```python
from build123d import *

# Parameters (mm, degrees)
BASE_DEPTH                   = 6.35
SUPPORT_CUTOUTS_REACH        = 181.717
SKETCH4_W                    = 12.7
SKETCH4_H                    = 6.35
SUPPORT_CUTOUT_PATTERN_COUNT = 4
F_8_CLEARANCE_HOLE1_D        = 4.4958
CABLE_HOLES_REACH            = 181.717
SKETCH14_R                   = 7.9375
ALIGNER_MOUNTING_HOLES_D     = 4.3053
CIRPATTERN1_COUNT            = 4
CUT_EXTRUDE2_DEPTH           = 180.717340566
CUT_EXTRUDE3_DEPTH           = 180.717340566


with BuildPart() as part:
    # Base sketch → Base (new body)
    with BuildSketch(Plane(origin=(0, 0, 0), x_dir=(1, 0, 0), z_dir=(0, 1, 0))):
        Polygon((-127, 52.605122421), (-127, -52.605122421), (-52.605122421, -127), (52.605122421, -127), (127, -52.605122421), (127, 52.605122421), (52.605122421, 127), (-52.605122421, 127), align=None)
    extrude(amount=BASE_DEPTH)

    # Sketch4 → Support cutouts (cut, up to next)
    with BuildSketch(Plane(origin=(0, 6.35, 0), x_dir=(1, 0, 0), z_dir=(0, 1, 0)), mode=Mode.PRIVATE) as support_cutouts_sk1:
        with Locations((0, 73.025)):
            Rectangle(SKETCH4_W, SKETCH4_H)
    support_cutouts_tool1 = extrude(support_cutouts_sk1.sketch, amount=-SUPPORT_CUTOUTS_REACH, mode=Mode.PRIVATE) & part.part
    support_cutouts = support_cutouts_tool1.solids().sort_by_distance((0, 6.35, -73.025))[0]
    add(support_cutouts, mode=Mode.SUBTRACT)

    # Support cutout pattern: Support cutouts ×4 about axis
    support_cutout_pattern_axis = Axis((0, 0, 0), (0, 1, 0))
    for i in range(1, SUPPORT_CUTOUT_PATTERN_COUNT):
        add(support_cutouts.rotate(support_cutout_pattern_axis, i * 360 / SUPPORT_CUTOUT_PATTERN_COUNT), mode=Mode.SUBTRACT)

    # 8 Clearance Hole1 (through all)
    with Locations(Plane(origin=(0, 6.35, 0), x_dir=(1, 0, 0), z_dir=(0, 1, 0))):
        with Locations((-82.55, 34.193329574), (-34.193329574, 82.55), (34.193329574, 82.55), (82.55, 34.193329574), (82.55, -34.193329574), (34.193329574, -82.55), (-34.193329574, -82.55), (-82.55, -34.193329574)):
            Hole(F_8_CLEARANCE_HOLE1_D / 2)

    # Sketch14 → Cable holes (cut, up to next)
    with BuildSketch(Plane(origin=(0, 6.35, 0), x_dir=(1, 0, 0), z_dir=(0, 1, 0)), mode=Mode.PRIVATE) as cable_holes_sk1:
        with Locations(Location((-53.881536726, 53.881536726, 0), (0, 0, 270))):
            Circle(SKETCH14_R)
    cable_holes_tool1 = extrude(cable_holes_sk1.sketch, amount=-CABLE_HOLES_REACH, mode=Mode.PRIVATE) & part.part
    # Sketch14 → Cable holes (cut, up to next)
    with BuildSketch(Plane(origin=(0, 6.35, 0), x_dir=(1, 0, 0), z_dir=(0, 1, 0)), mode=Mode.PRIVATE) as cable_holes_sk2:
        with Locations(Location((53.881536726, 53.881536726, 0), (0, 0, 270))):
            Circle(SKETCH14_R)
    cable_holes_tool2 = extrude(cable_holes_sk2.sketch, amount=-CABLE_HOLES_REACH, mode=Mode.PRIVATE) & part.part
    # Sketch14 → Cable holes (cut, up to next)
    with BuildSketch(Plane(origin=(0, 6.35, 0), x_dir=(1, 0, 0), z_dir=(0, 1, 0)), mode=Mode.PRIVATE) as cable_holes_sk3:
        with Locations(Location((53.881536726, -53.881536726, 0), (0, 0, 270))):
            Circle(SKETCH14_R)
    cable_holes_tool3 = extrude(cable_holes_sk3.sketch, amount=-CABLE_HOLES_REACH, mode=Mode.PRIVATE) & part.part
    # Sketch14 → Cable holes (cut, up to next)
    with BuildSketch(Plane(origin=(0, 6.35, 0), x_dir=(1, 0, 0), z_dir=(0, 1, 0)), mode=Mode.PRIVATE) as cable_holes_sk4:
        with Locations(Location((-53.881536726, -53.881536726, 0), (0, 0, 270))):
            Circle(SKETCH14_R)
    cable_holes_tool4 = extrude(cable_holes_sk4.sketch, amount=-CABLE_HOLES_REACH, mode=Mode.PRIVATE) & part.part
    add(cable_holes_tool1.solids().sort_by_distance((-53.881537, 6.35, -53.881537))[0], mode=Mode.SUBTRACT)
    add(cable_holes_tool2.solids().sort_by_distance((53.881537, 6.35, -53.881537))[0], mode=Mode.SUBTRACT)
    add(cable_holes_tool3.solids().sort_by_distance((53.881537, 6.35, 53.881537))[0], mode=Mode.SUBTRACT)
    add(cable_holes_tool4.solids().sort_by_distance((-53.881537, 6.35, 53.881537))[0], mode=Mode.SUBTRACT)

    # aligner mounting holes (through all)
    with Locations(Plane(origin=(0, 6.35, 0), x_dir=(1, 0, 0), z_dir=(0, 1, 0))):
        with Locations((121.233457634, 40.411152545), (40.411152545, 121.233457634)):
            aligner_mounting_holes = Hole(ALIGNER_MOUNTING_HOLES_D / 2)

    # CirPattern1: aligner mounting holes ×4 about axis
    cirpattern1_axis = Axis((0, 0, 0), (0, 1, 0))
    for i in range(1, CIRPATTERN1_COUNT):
        add(aligner_mounting_holes.rotate(cirpattern1_axis, i * 360 / CIRPATTERN1_COUNT), mode=Mode.SUBTRACT)

    # Sketch28 → Cut-Extrude2 (cut, through all)
    with BuildSketch(Plane(origin=(0, 6.35, 0), x_dir=(1, 0, 0), z_dir=(0, 1, 0))):
        with BuildLine():
            Line((55.651152545, 80.367817332), (55.651152545, 107.308585695))
            ThreePointArc((55.651152545, 107.308585695), (57.611132647, 110.241903211), (61.071216575, 109.553649725))
            Line((61.071216575, 109.553649725), (109.553649725, 61.071216575))
            ThreePointArc((109.553649725, 61.071216575), (110.241903211, 57.611132647), (107.308585695, 55.651152545))
            Line((107.308585695, 55.651152545), (80.367817332, 55.651152545))
            ThreePointArc((80.367817332, 55.651152545), (79.152797434, 55.892835029), (78.122753301, 56.581088515))
            Line((78.122753301, 56.581088515), (56.581088515, 78.122753301))
            ThreePointArc((56.581088515, 78.122753301), (55.892835029, 79.152797434), (55.651152545, 80.367817332))
        make_face()
        with BuildLine():
            Line((80.367817332, -55.651152545), (107.308585695, -55.651152545))
            ThreePointArc((107.308585695, -55.651152545), (110.241903211, -57.611132647), (109.553649725, -61.071216575))
            Line((109.553649725, -61.071216575), (61.071216575, -109.553649725))
            ThreePointArc((61.071216575, -109.553649725), (57.611132647, -110.241903211), (55.651152545, -107.308585695))
            Line((55.651152545, -107.308585695), (55.651152545, -80.367817332))
            ThreePointArc((55.651152545, -80.367817332), (55.892835029, -79.152797434), (56.581088515, -78.122753301))
            Line((56.581088515, -78.122753301), (78.122753301, -56.581088515))
            ThreePointArc((78.122753301, -56.581088515), (79.152797434, -55.892835029), (80.367817332, -55.651152545))
        make_face()
        with BuildLine():
            Line((-55.651152545, -80.367817332), (-55.651152545, -107.308585695))
            ThreePointArc((-55.651152545, -107.308585695), (-57.611132647, -110.241903211), (-61.071216575, -109.553649725))
            Line((-61.071216575, -109.553649725), (-109.553649725, -61.071216575))
            ThreePointArc((-109.553649725, -61.071216575), (-110.241903211, -57.611132647), (-107.308585695, -55.651152545))
            Line((-107.308585695, -55.651152545), (-80.367817332, -55.651152545))
            ThreePointArc((-80.367817332, -55.651152545), (-79.152797434, -55.892835029), (-78.122753301, -56.581088515))
            Line((-78.122753301, -56.581088515), (-56.581088515, -78.122753301))
            ThreePointArc((-56.581088515, -78.122753301), (-55.892835029, -79.152797434), (-55.651152545, -80.367817332))
        make_face()
        with BuildLine():
            Line((-56.581088515, 78.122753301), (-78.122753301, 56.581088515))
            ThreePointArc((-78.122753301, 56.581088515), (-79.152797434, 55.892835029), (-80.367817332, 55.651152545))
            Line((-80.367817332, 55.651152545), (-107.308585695, 55.651152545))
            ThreePointArc((-107.308585695, 55.651152545), (-110.241903211, 57.611132647), (-109.553649725, 61.071216575))
            Line((-109.553649725, 61.071216575), (-61.071216575, 109.553649725))
            ThreePointArc((-61.071216575, 109.553649725), (-57.611132647, 110.241903211), (-55.651152545, 107.308585695))
            Line((-55.651152545, 107.308585695), (-55.651152545, 80.367817332))
            ThreePointArc((-55.651152545, 80.367817332), (-55.892835029, 79.152797434), (-56.581088515, 78.122753301))
        make_face()
    extrude(amount=-CUT_EXTRUDE2_DEPTH, mode=Mode.SUBTRACT)

    # Sketch29 → Cut-Extrude3 (cut, through all)
    with BuildSketch(Plane(origin=(0, 6.35, 0), x_dir=(1, 0, 0), z_dir=(0, 1, 0))):
        with BuildLine():
            Line((15.24, -2.2225), (15.24, 2.2225))
            ThreePointArc((15.24, 2.2225), (15.983948776, 4.018551224), (17.78, 4.7625))
            Line((17.78, 4.7625), (19.05, 4.7625))
            ThreePointArc((19.05, 4.7625), (20.846051224, 4.018551224), (21.59, 2.2225))
            Line((21.59, 2.2225), (21.59, -2.2225))
            ThreePointArc((21.59, -2.2225), (20.846051224, -4.018551224), (19.05, -4.7625))
            Line((19.05, -4.7625), (17.78, -4.7625))
            ThreePointArc((17.78, -4.7625), (15.983948776, -4.018551224), (15.24, -2.2225))
        make_face()
        with BuildLine():
            Line((2.2225, 15.24), (-2.2225, 15.24))
            ThreePointArc((-2.2225, 15.24), (-4.018551224, 15.983948776), (-4.7625, 17.78))
            Line((-4.7625, 17.78), (-4.7625, 19.05))
            ThreePointArc((-4.7625, 19.05), (-4.018551224, 20.846051224), (-2.2225, 21.59))
            Line((-2.2225, 21.59), (2.2225, 21.59))
            ThreePointArc((2.2225, 21.59), (4.018551224, 20.846051224), (4.7625, 19.05))
            Line((4.7625, 19.05), (4.7625, 17.78))
            ThreePointArc((4.7625, 17.78), (4.018551224, 15.983948776), (2.2225, 15.24))
        make_face()
        with BuildLine():
            Line((-2.2225, -15.24), (2.2225, -15.24))
            ThreePointArc((2.2225, -15.24), (4.018551224, -15.983948776), (4.7625, -17.78))
            Line((4.7625, -17.78), (4.7625, -19.05))
            ThreePointArc((4.7625, -19.05), (4.018551224, -20.846051224), (2.2225, -21.59))
            Line((2.2225, -21.59), (-2.2225, -21.59))
            ThreePointArc((-2.2225, -21.59), (-4.018551224, -20.846051224), (-4.7625, -19.05))
            Line((-4.7625, -19.05), (-4.7625, -17.78))
            ThreePointArc((-4.7625, -17.78), (-4.018551224, -15.983948776), (-2.2225, -15.24))
        make_face()
        with BuildLine():
            Line((-15.24, 2.2225), (-15.24, -2.2225))
            ThreePointArc((-15.24, -2.2225), (-15.983948776, -4.018551224), (-17.78, -4.7625))
            Line((-17.78, -4.7625), (-19.05, -4.7625))
            ThreePointArc((-19.05, -4.7625), (-20.846051224, -4.018551224), (-21.59, -2.2225))
            Line((-21.59, -2.2225), (-21.59, 2.2225))
            ThreePointArc((-21.59, 2.2225), (-20.846051224, 4.018551224), (-19.05, 4.7625))
            Line((-19.05, 4.7625), (-17.78, 4.7625))
            ThreePointArc((-17.78, 4.7625), (-15.983948776, 4.018551224), (-15.24, 2.2225))
        make_face()
    extrude(amount=-CUT_EXTRUDE3_DEPTH, mode=Mode.SUBTRACT)


solid = part.part
```
Geometry check sheet. Reference: the model listing, model coordinates, mm. A direction names the side the tool comes from. Round coordinates to 2 decimals unless told otherwise and drop trailing zeros. Order: outer loops, then holes, each group sorted by start corner. A loop starts at its lowest first (then second) coordinate and runs counter-clockwise, first axis right, second up. Notation, with made-up numbers: (34, 46.5) - (42, 46.5) arc R11 ccw to (42, 67.5) - close; hole circle Ø5 at (83, 51.5). An arc over 180 degrees is marked (long way). Use a Markdown table: item, result. Add a question column.
1) Gauge pin test, flat ends, axial feed: P1, Ø1.9, axis at x = -71.5, y = 3.5, coming from the +Z side; P2, Ø1, axis at x = 77, y = 4, coming from the -Z side; P3, Ø1.9, axis at y = 4, z = -73, coming from the +X side. Record the tip position at first contact, or that the pin passes through.
2) Section check B-B (y = 3.75). Count the separate pieces of the cut face and the enclosed holes in it, then the cut area to 3 significant figures.
3) Mould release check, pull along X, two halves, no side actions. Record for faces 1 (the flat face through (-6.35, 3, 73)), 2 (the flat face through (90.323, 3.131, -89.282)), 3 (the flat face through (84.973, 3.219, -85.652)): released by +X, released by -X, zero draft, split by the parting line, or undercut.
4) Set-up check for faces 4 (the flat face through (89.282, 3.131, 90.323)), 5 (the flat face through (0, 3, 76.2)): record each of +Z, -Z, +X, -X, +Y, -Y from which the full face is reachable in a straight line by a thin tool's end or side.
5) Thickness scan on line 1 along Z through (x, y) = (6, 1); line 2 along Z through (x, y) = (1, 0.75); line 3 along X through (y, z) = (3.5, 70.5). Record the ranges inside material, lowest first.
6) Section check A-A (x = -95). Record the cut outline in (y, z), then the cut area to 3 significant figures.
Established:
| question | item | result |
|---|---|---|
| 1 | P1 | z = 109.06 |
| 1 | P2 | z = -103.11 |
| 1 | P3 | x = 107.56 |
| 2 | separate pieces | 1 |
| 2 | enclosed holes | 32 |
| 2 | area | 46,000 mm2 |
| 3 | face 1 | undercut |
| 3 | face 2 | released by +X |
| 3 | face 3 | undercut |
| 4 | face 4 | +Z, +X, +Y, -Y |
| 4 | face 5 | +Y, -Y |
| 5 | line 1 | -127 to -76.2, -69.85 to 69.85, 76.2 to 127 |
| 5 | line 2 | -127 to -76.2, -69.85 to -21.59, -15.24 to 15.24, 21.59 to 69.85, 76.2 to 127 |
| 5 | line 3 | -109.11 to -100.12, -64.2 to -6.35, 6.35 to 64.2, 100.12 to 109.11 |
| 6 | outline | (0, -84.61) - (6.35, -84.61) - (6.35, -75.62) - (0, -75.62) - close; (0, -55.65) - (6.35, -55.65) - (6.35, 55.65) - (0, 55.65) - close; (0, 75.62) - (6.35, 75.62) - (6.35, 84.61) - (0, 84.61) - close |
| 6 | area | 821 mm2 |
